Part print with two shaded views. Sizes in mm from the minimum x, y, z corner. Round coordinates to 2 decimals unless told otherwise and drop trailing zeros. Order: outer loops, then holes, each group sorted by start corner. A loop starts at its lowest first (then second) coordinate and runs counter-clockwise, first axis right, second up. Notation, with made-up numbers: M -7,81 L 29,81 A29 ccw 29,119 Z; hole C -17.5,28 d6. An arc over 180 degrees is marked long. Return JSON: item names as keys, results as strings. Group by question number.
Item 1: Probe line 1 along X through (y, z) = (13.5, 29.5); line 2 along Z through (x, y) = (30, 10); line 3 along Z through (x, y) = (47.5, 27.5). List the from-to ranges inside material, lowest first.
Item 2: Pin check, flat tips, straight feed: pin 1 Ø4 at (x, y) = (9.5, 20.5) entering from -Z; pin 2 Ø5 at (y, z) = (13.5, 53) entering from -X; pin 3 Ø1 at (y, z) = (6.5, 45) entering from +X. Stop position of each tip, or through.
Item 3: Slice it at B-B on x = 30. Write the cut outline in (y, z), then the cut area to 3 significant figures.
Item 4: Slice it at A-A on z = 30. Write the cut outline in (x, y), then the cut area to 3 significant figures.
Item 5: Slice it at C-C on y = 2.5. Write the cut outline in (x, z), then the cut area to 3 significant figures.
Item 6: Slice it at D-D on x = 9. Write the cut outline in (y, z), then the cut area to 3 significant figures.
Item 7: Pull direction Z, two halves, no side cores. Call the marked faces 1, 2, 3 and 4: pulls with the +Z half, pulls with the -Z half, needs draft (parallel to the pull), parting line crosses it, or undercut.
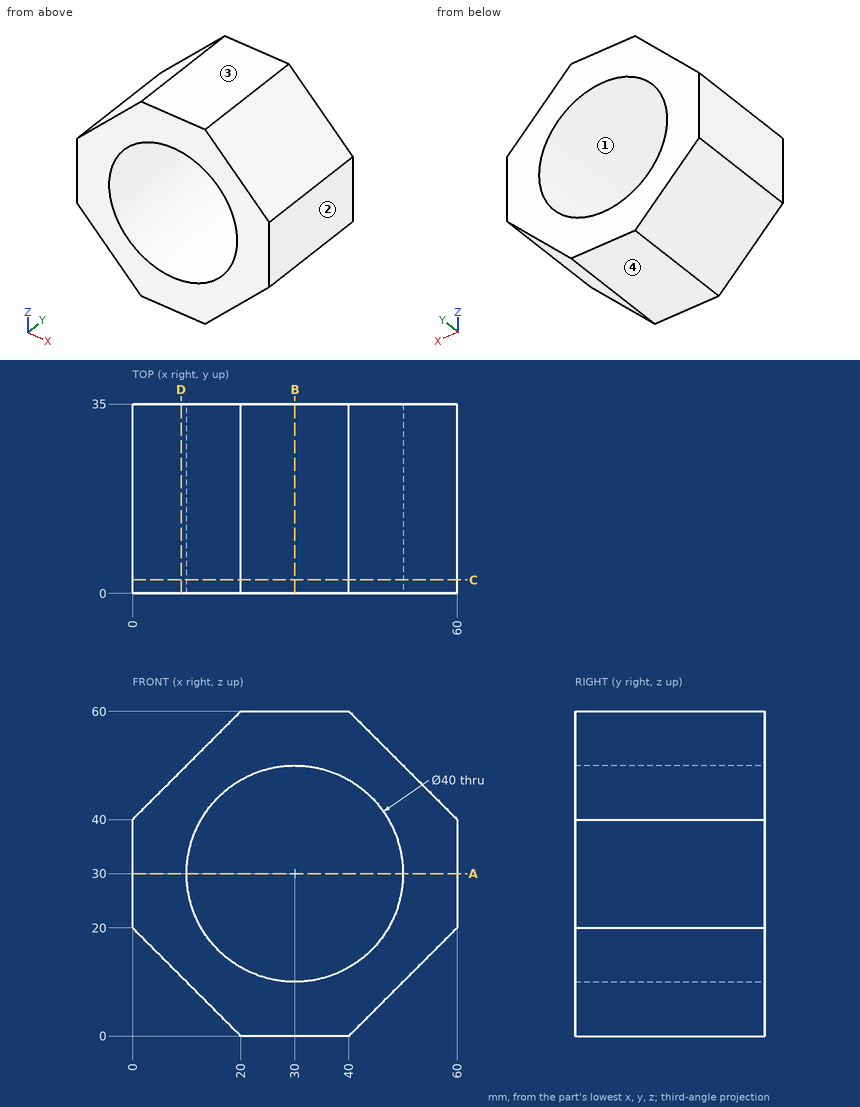
Output values:
{
 "1": {"line 1": "0 to 10.01, 49.99 to 60", "line 2": "0 to 10, 50 to 60", "line 3": "7.5 to 20.32, 39.68 to 52.5"},
 "2": {"pin 1": "z = 8.5", "pin 2": "x = 10.5", "pin 3": "x = 55.5"},
 "3": {"outline": "M 0,0 L 35,0 L 35,10 L 0,10 Z; M 0,50 L 35,50 L 35,60 L 0,60 Z", "area": "700 mm²"},
 "4": {"outline": "M 0,0 L 10,0 L 10,35 L 0,35 Z; M 50,0 L 60,0 L 60,35 L 50,35 Z", "area": "700 mm²"},
 "5": {"outline": "M 0,20 L 20,0 L 40,0 L 60,20 L 60,40 L 40,60 L 20,60 L 0,40 Z; hole C 30,30 d40", "area": "1,540 mm²"},
 "6": {"outline": "M 0,11 L 35,11 L 35,49 L 0,49 Z", "area": "1,330 mm²"},
 "7": {"face 1": "undercut", "face 2": "needs draft", "face 3": "pulls with the +Z half", "face 4": "pulls with the -Z half"}
}
